Autodesk Inventor part; units mm, degrees
ref_plane "YZ Plane" through (0, 0, 0) normal (1, 0, 0) x (0, 1, 0)
ref_plane "XZ Plane" through (0, 0, 0) normal (0, 1, 0) x (-1, 0, 0)
ref_plane "XY Plane" through (0, 0, 0) normal (0, 0, 1) x (1, 0, 0)
sketch "Sketch2" plane through (0, 0, 0) normal (0, 1, 0) x (-1, 0, 0)
  line L0 (3.9324, 0) -> (5, 0)
  arc A0 (3.9324, 0) -> (1.9324, -2) centre (3.9324, -2) ccw
  line L1 (3.9324, 0) -> (6.9065, 0)
  line L2 (3.9324, 0) -> (6.3389, 0)
  arc A1 (7.9907, -0.8725) -> (36.874, -0.8725) centre (22.4324, 8.9853) ccw
  line L3 (38.5258, 0) -> (57.6864, 0)
  arc A2 (71.4324, 0) -> (59.6229, 1.5) centre (65.4324, 0) ccw
  circle A3 centre (65.4324, 0) radius 1.5
  arc A4 (57.6864, 0) -> (59.6229, 1.5) centre (57.6864, 2) ccw
  arc A5 (38.5258, 0) -> (36.874, -0.8725) centre (38.5258, -2) ccw
  arc A6 (7.9907, -0.8725) -> (6.3389, 0) centre (6.3389, -2) ccw
  arc A7 (59.3504, -1.7983) -> (57.1879, 0) centre (57.1879, -2.1995) ccw
  line L4 (77.1831, 8.9853) -> (-10.6505, 8.9853) construction
  line L5 (3.9324, 17.9706) -> (5, 17.9706)
  arc A8 (42.998, 40.9699) -> (1.9324, 19.9706) centre (55.0831, -33.3161) ccw
  arc A9 (1.9324, 19.9706) -> (3.9324, 17.9706) centre (3.9324, 19.9706) ccw
  line L6 (3.9324, 17.9706) -> (6.9065, 17.9706)
  line L7 (3.9324, 17.9706) -> (6.3389, 17.9706)
  arc A10 (36.874, 18.843) -> (7.9907, 18.843) centre (22.4324, 8.9853) ccw
  line L8 (38.5258, 17.9706) -> (57.6864, 17.9706)
  arc A11 (59.6229, 16.4706) -> (71.4324, 17.9706) centre (65.4324, 17.9706) ccw
  arc A12 (71.4324, 17.9706) -> (42.998, 40.9699) centre (43.4479, 12.4496) ccw
  circle A13 centre (65.4324, 17.9706) radius 1.5
  arc A14 (59.6229, 16.4706) -> (57.6864, 17.9706) centre (57.6864, 15.9706) ccw
  arc A15 (36.874, 18.843) -> (38.5258, 17.9706) centre (38.5258, 19.9706) ccw
  arc A16 (6.3389, 17.9706) -> (7.9907, 18.843) centre (6.3389, 19.9706) ccw
  arc A17 (65.6797, 24.421) -> (59.3504, 19.7689) centre (64.5387, 19.3419) ccw
  arc A18 (65.6797, 24.421) -> (67.6049, 27.617) centre (65.5936, 26.6507) ccw
  arc A19 (57.1879, 17.9706) -> (59.3504, 19.7689) centre (57.1879, 20.1701) ccw
  line L9 (1.9324, -2) -> (1.9324, -12)
  line L10 (3.9324, -14) -> (69.4324, -14)
  arc A20 (1.9324, -12) -> (3.9324, -14) centre (3.9324, -12) ccw
  line L11 (71.4324, 0) -> (71.4324, -12)
  arc A21 (69.4324, -14) -> (71.4324, -12) centre (69.4324, -12) ccw
  arc A22 (59.3504, -1.7983) -> (71.4324, -2.4583) centre (65.4715, -0.6626) ccw
  point P0 (0, 0)
  point P1 (7.4324, 0)
  point P2 (37.4324, 0)
  point P3 (22.4324, -8.5)
  point P4 (0, 17.9706)
  point P5 (7.4324, 17.9706)
  point P6 (37.4324, 17.9706)
  point P7 (22.4324, 26.4706)
  point P8 (71.4324, 17.9706)
  point P9 (6.3389, 17.9706)
  dimension "d3" = 2
  dimension "d12" = 3.5
  dimension "d13" = 30
  dimension "d14" = 8.5
  dimension "d17" = 3
  dimension "d18" = 2
  dimension "d19" = 2
  dimension "d21" = 0
  dimension "d22" = 0
  dimension "d91" = 3.9324
  dimension "d92" = 2
  dimension "d93" = 28
  dimension "d94" = 2
  dimension "d107" = 10
extrude "Extrusion1" add sketch "Sketch2" along normal mid plane 30 contours L0 L1 A6 A1 A5 L3 A7 A22 L11 A21 L10 A20 L9 A0 | L3 A4 A2 L11 A22 A7
extrude "Extrusion2" cut sketch "Sketch2" along normal mid plane 15 contours L3 A4 A2 L11 A22 A7
sketch "Sketch7" plane through (0, -15, 0) normal (0, -1, 0) x (1, 0, 0)
  arc A0 (-6.3389, 0) -> (-7.9907, -0.8725) centre (-6.3389, -2) ccw
  line L0 (-7.9907, -0.8725) -> (-7.9907, -1.8725)
  arc A1 (-36.874, -0.8725) -> (-7.9907, -0.8725) centre (-22.4324, 8.9853) ccw
  line L1 (-36.874, -0.8725) -> (-36.874, -1.8725)
  arc A2 (-36.874, -1.8725) -> (-7.9907, -1.8725) centre (-22.4324, 8.9853) ccw
  point P0 (0, 0)
  dimension "d59" = 1
  dimension "d60" = 1
extrude "Extrusion10" cut sketch "Sketch7" against normal up to next
fillet "Fillet4" radius 2 1 edges at (-71.4324, 0, -2.4583)
sketch "Sketch13" plane through (-57.6864, -15, 0) normal (0, 0, 1) x (1, 0, 0)
  circle A0 centre (10.6864, 15) radius 4
  line L0 (55.754, 30) -> (55.754, 0)
  point P0 (57.6864, 15)
  dimension "d99" = 8
  dimension "d106" = 47
extrude "Extrusion15" cut sketch "Sketch13" against normal up to next
sketch "Sketch14" plane through (-3.9324, 15, -14) normal (0, 0, -1) x (-1, 0, 0)
  circle A0 centre (43.0676, -15) radius 4
  line L0 (43.0676, -21.3509) -> (37.5676, -18.1754)
  line L1 (37.5676, -18.1754) -> (37.5676, -11.8246)
  line L2 (37.5676, -11.8246) -> (43.0676, -8.6491)
  line L3 (43.0676, -8.6491) -> (48.5676, -11.8246)
  line L4 (48.5676, -11.8246) -> (48.5676, -18.1754)
  line L5 (48.5676, -18.1754) -> (43.0676, -21.3509)
  line L6 (67.5, -30) -> (67.5, 0)
  point P0 (-3.9324, -15)
  point P1 (37.5676, -15)
  dimension "d103" = 11
extrude "Extrusion16" cut sketch "Sketch14" against normal blind 2
sketch "Sketch15" plane through (-3.9324, 15, -14) normal (0, 0, -1) x (-1, 0, 0)
  line L0 (32.6944, -26.5) -> (-17.3056, -26.5)
  line L1 (-17.3056, -26.5) -> (-17.3056, -3.5)
  line L2 (-17.3056, -3.5) -> (32.6944, -3.5)
  line L3 (32.6944, -3.5) -> (32.6944, -26.5)
  line L4 (0, 0) -> (65.5, 0)
  line L5 (32.9416, -30) -> (4.0584, -30)
  line L6 (-17.3056, -26.5) -> (32.75, -26.5)
  line L7 (32.75, -26.5) -> (32.75, -30)
  line L8 (32.75, -30) -> (-17.3056, -30)
  line L9 (-17.3056, -30) -> (-17.3056, -26.5)
  point P0 (7.6944, -26.5)
  point P1 (4.0584, -30)
  dimension "d111" = 50
  dimension "d112" = 23
extrude "Extrusion17" add sketch "Sketch15" along normal blind 20
sketch "Sketch17" plane through (-3.9324, 15, -34) normal (0, 0, -1) x (-1, 0, 0)
  line L0 (-17.3056, -26.5) -> (32.75, -26.5)
  line L1 (32.75, -30) -> (-17.3056, -30)
  line L2 (32.6944, -26.5) -> (-17.3056, -26.5)
  line L3 (-17.3056, -3.5) -> (32.6944, -3.5)
  circle A0 centre (-12.8056, -23.5) radius 1
  line L4 (-17.3056, -26.5) -> (-17.3056, -3.5)
  line L5 (-17.3056, -30) -> (-17.3056, -26.5)
  circle A1 centre (-5.3045, -15.2368) radius 8
  circle A2 centre (20.6944, -15) radius 8
  line L6 (32.75, -26.5) -> (32.75, -30)
  line L7 (32.9416, -30) -> (4.0584, -30)
  line L8 (32.6944, -3.5) -> (32.6944, -26.5)
  circle A3 centre (28.1944, -7) radius 1
  point P0 (-3.9324, -15)
  point P1 (-3.9324, -15)
  point P2 (7.6944, -26.5)
  point P3 (-3.9324, -15)
  point P4 (0, 0)
  point P5 (7.6944, -13.0925)
  dimension "d142" = 50
  dimension "d143" = 23
  dimension "d144" = 25
  dimension "d145" = 2
  dimension "d146" = 2
  dimension "d147" = 41
  dimension "d148" = 16.5
  dimension "d149" = 3.5
  dimension "d150" = 4.5
  dimension "d151" = 16
  dimension "d152" = 16
  dimension "d153" = 26
  dimension "d154" = 11.5
  dimension "d155" = 13
extrude "Extrusion18" cut sketch "Sketch17" against normal blind 2 contours A0 | A1 | A2 | A3
sketch "Sketch18" plane through (-3.9324, 11.5, -14) normal (0, 1, 0) x (1, 0, 0)
  line L0 (-30.6944, 2) -> (15.3056, 2)
  line L1 (15.3056, 2) -> (15.3056, 18)
  line L2 (15.3056, 18) -> (-30.6944, 18)
  line L3 (-30.6944, 18) -> (-30.6944, 2)
  line L4 (-32.6944, 20) -> (17.3056, 20)
  line L5 (0, 0) -> (-65.5, 0)
  line L6 (17.3056, 0) -> (17.3056, 20)
  line L7 (-32.6944, 0) -> (-32.6944, 20)
  point P0 (3.9324, -14)
  dimension "d158" = 2
  dimension "d159" = 2
  dimension "d160" = 2
  dimension "d161" = 2
extrude "Extrusion19" cut sketch "Sketch18" against normal blind 21
sketch "Sketch19" plane through (-3.9324, -9.5, -14) normal (0, 1, 0) x (1, 0, 0)
  line L0 (-30.6944, 18) -> (12.8056, 18)
  line L1 (-15.6944, 6) -> (0.3056, 6)
  line L2 (0.3056, 6) -> (0.3056, 18)
  line L3 (0.3056, 18) -> (-15.6944, 18)
  line L4 (-15.6944, 18) -> (-15.6944, 6)
  line L5 (-30.6944, 2) -> (-30.6944, 18)
  point P0 (3.9324, -14)
  point P1 (-15.6944, 18)
  dimension "d164" = 15
  dimension "d165" = 16
  dimension "d168" = 12
extrude "Extrusion20" cut sketch "Sketch19" against normal blind 20
properties part number "Bike_Mount_Right"
Here's how the part is built. I have some questions about the finished solid (model axes, mm). A direction names the side the tool comes from. Coordinates: 2 decimals unless noted, no trailing zeros. Order: outer loops, then holes, each group sorted by start corner. A loop starts at its lowest first (then second) coordinate and runs counter-clockwise, first axis right, second up. Notation, with made-up numbers: M 4.5,-25.5 L 57.5,-25.5 A31 ccw 57.5,1.5 Z; hole C -33.5,59 d3. An arc over 180 degrees is marked long. Answer as a JSON object with one key per item and string values. Group by question number.
(1) Suppose I cut it at A-A, the plane z = -27. Please give me the cut outline in (x, y).
(2) Suppose I cut it at B-B, the plane y = 10. Please give me the cut outline in (x, z), then the cut area to 3 significant figures.
(3) I need wall thicknesses on probe 1 along X at (y, z) = (3.25, -26.5); probe 2 along Z at (x, y) = (6, 6.75); probe 3 along Z at (x, y) = (-48, 7). Which ranges of each line are inside material? Lowest first, please.
(4) Suppose I cut it at D-D, the plane x = -28. Please give me the cut outline in (y, z).
(5) If we mould it in two halves opening along Z, with no side actions, what happens to faces 1 (the face through (-62.881, -0.105, -6.323)), 2 (the face through (13.373, -2, -24)), 3 (the face through (-19.627, -12, -26))? For each: released by +Z, released by -Z, zero draft, split by the parting line, or undercut.
(6) For pin 1 (9.5 mm diameter, centred on x = 1.37, y = -0.24, fed in from +Z); pin 2 (13 mm diameter, centred on x = -24.63, y = 0, fed in from -Z); pin 3 (1.6 mm diameter, centred on y = -12.5, z = -28, fed in from -X), each with a flat end and sliding along its axis, tell me the tip position at first contact or that it passes through.
(7) Which directions (+Z, -Z, +X, -X, +Y, -Y) give clear straight access to the entire face, cutting with the end or side of a thin tool? Please do faces 4 (the face through (-36.682, -13, -24)), 5 (the face through (-51, 6, -14)), 6 (the face through (-34.627, 1, -24)).
(8) Suppose I cut it at C-C, the plane x = 5.5. Please give me the cut outline in (y, z).
Values found:
{
 "1": {"outline": "M -36.68,-15 L -19.63,-15 L -19.63,-9.5 L -34.63,-9.5 L -34.63,11.5 L -36.63,11.5 L -36.63,-11.5 L -36.68,-11.5 Z; M -3.63,-15 L 13.37,-15 L 13.37,11.5 L 11.37,11.5 L 11.37,-9.5 L -3.63,-9.5 Z"},
 "2": {"outline": "M -71.43,-12 A2 ccw -69.43,-14 L -36.63,-14 L -36.63,-34 L 13.37,-34 L 13.37,-14 L -3.93,-14 A2 ccw -1.93,-12 L -1.93,-2 A2 ccw -3.93,0 L -6.34,0 A2 ccw -7.99,-0.87 L -7.99,-1.87 A18.07 cw -36.87,-1.87 L -36.87,-0.87 A2 ccw -38.53,0 L -57.69,0 A2 cw -59.62,1.5 A6 ccw -71.43,0 Z; hole C -65.43,0 d3; hole M -34.63,-32 L 11.37,-32 L 11.37,-16 L -34.63,-16 Z", "area": "1,080 mm^2"},
 "3": {"probe 1": "x = -36.63 to -34.63, 11.37 to 13.37", "probe 2": "z = -34 to -32, -16 to -14", "probe 3": "z = -14 to 0"},
 "4": {"outline": "M -15,-34 L -7.25,-34 L -7.25,-32 L -9.5,-32 L -9.5,-16 L 11.5,-16 L 11.5,-14 L 15,-14 L 15,-8.2 L -15,-8.2 Z; M 7.25,-34 L 11.5,-34 L 11.5,-32 L 7.25,-32 Z"},
 "5": {"face 1": "released by +Z", "face 2": "zero draft", "face 3": "undercut"},
 "6": {"pin 1": "stops at z = -0.08", "pin 2": "stops at z = -16", "pin 3": "stops at x = -36.68"},
 "7": {"face 4": "-Z, -X, +Y, -Y", "face 5": "-Z, -X, +Y", "face 6": "+Y"},
 "8": {"outline": "M -15,-34 L -7.09,-34 L -7.09,-32 L -9.5,-32 L -9.5,-16 L 11.5,-16 L 11.5,-14 L -15,-14 Z; M 6.62,-34 L 11.5,-34 L 11.5,-32 L 6.62,-32 Z"}
}
